The figure shows three views and two pictorial views of one solid part (mm, origin at its lowest corner). Answer the questions. A direction names the side the tool comes from. Give positions to 0.01 mm unless a question says otherwise; leave off trailing zeros. Order: outer loops, then holes, each group sorted by start corner. A loop starts at its lowest first (then second) coordinate and runs counter-clockwise, first axis right, second up. Notation, with made-up numbers: (-4, 52) - (51, 52) arc R27 cw to (51, 69) - close; hole circle Ø8 at (-29, 51.25). An arc over 180 degrees is marked (long way). Use a Markdown table: item, result. Add a question column.
1. Flat-ended cylindrical pins translate along their axes: P1, Ø0.5, axis at x = 6.5, z = 3, coming from the +Y side; P2, Ø2, axis at y = 8, z = 2.5, coming from the +X side. Find the tip coordinate at first contact, or state that the pin passes through.
2. A cutting plane is placed at B-B on z = 0.55. Determine the outline of the cut face in (x, y).
3. A cutting plane is placed at C-C on y = 3. Determine the outline of the cut face in (x, z), and give its area (3 significant figures).
4. Which of the six approach directions +Z, -Z, +X, -X, +Y, -Y give full straight-line access (tool end or side, diameter ignored) to the marked faces 4, 5 and 6?
5. Consider L1, parallel to Y at x = 1.75, z = 2.15; L2, parallel to X at y = 5.25, z = 0.7; L3, parallel to X at y = 7.25, z = 0.6. Determine where each line is inside the solid, lowest interval first.
6. For a pull along Y with two mould halves and no side action, classify the marked faces 1, 2 and 3 as released by +Y, released by -Y, zero draft, split by the parting line, or undercut.
7. A cutting plane is placed at D-D on y = 7.5. Determine the outline of the cut face in (x, z), and give its area (3 significant figures).
8. A cutting plane is placed at A-A on x = 3.25. Determine the outline of the cut face in (y, z).
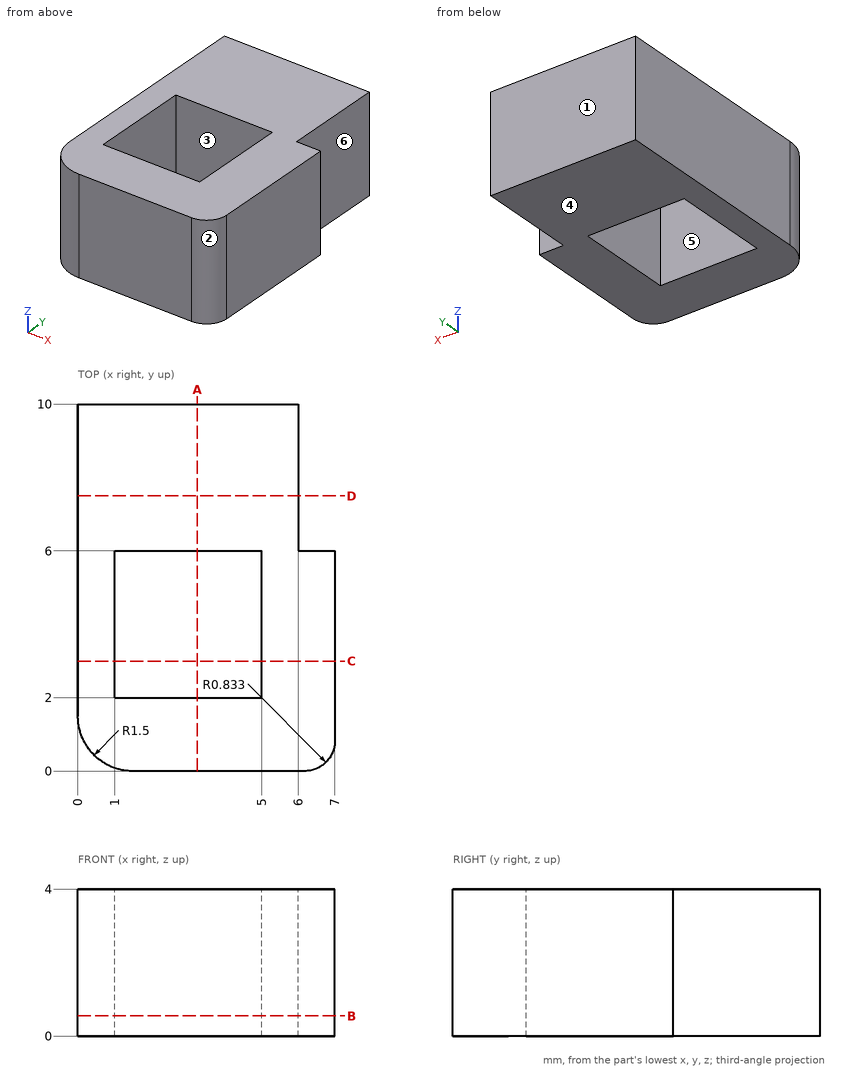
Output values:
| question | item | result |
|---|---|---|
| 1 | P1 | y = 6 |
| 1 | P2 | x = 6 |
| 2 | outline | (0, 1.5) arc R1.5 ccw to (1.5, 0) - (6.17, 0) arc R0.83 ccw to (7, 0.83) - (7, 6) - (6, 6) - (6, 10) - (0, 10) - close; hole (1, 2) - (5, 2) - (5, 6) - (1, 6) - close |
| 3 | outline | (0, 0) - (1, 0) - (1, 4) - (0, 4) - close; (5, 0) - (7, 0) - (7, 4) - (5, 4) - close |
| 3 | area | 12.0 mm² |
| 4 | face 4 | -Z, +X, -X, +Y, -Y |
| 4 | face 5 | +Z, -Z |
| 4 | face 6 | +Z, -Z, +X, +Y |
| 5 | L1 | 0 to 2, 6 to 10 |
| 5 | L2 | 0 to 1, 5 to 7 |
| 5 | L3 | 0 to 6 |
| 6 | face 1 | released by +Y |
| 6 | face 2 | released by -Y |
| 6 | face 3 | undercut |
| 7 | outline | (0, 0) - (6, 0) - (6, 4) - (0, 4) - close |
| 7 | area | 24.0 mm² |
| 8 | outline | (0, 0) - (2, 0) - (2, 4) - (0, 4) - close; (6, 0) - (10, 0) - (10, 4) - (6, 4) - close |
